Here's how the part is built. I have some questions about the finished solid (model axes, mm). Round coordinates to 2 decimals unless told otherwise and drop trailing zeros. Write each loop counter-clockwise with the first axis right and the second up, starting at its lowest first coordinate (ties: lowest second). Pieces come first, ordered by that corner, then holes. Notation, with made-up numbers: M 54.25,45.25 L 67.25,45.25 A24 cw 67.25,56.25 Z; hole C 49,54.5 d11. An arc over 180 degrees is marked long. Use one line per item in the form item = value. Start each with the question number.
Q1. I want a section at A-A on y = -6. List the corners of the cut face in (x, z) for me, and give its area (3 significant figures).
Q2. I want a section at C-C on x = 16. List the corners of the cut face in (y, z) for me, and give its area (3 significant figures).
Q3. I need wall thicknesses on line 1 along X through (y, z) = (-15.25, 0.25); line 2 along X through (y, z) = (-5.5, 0.8). Which ranges of each line are inside material? Lowest first, please. Write a range as from..to.
Q4. I want a section at D-D on z = 0.3. State how many separate pieces and enclosed holes the cut face has, and give its area (3 significant figures).
Q5. I'm going to push a flat-ended pin straight in: pin 1 Ø2.5 at (x, y) = (15.25, 15.25) entering from +Z. Where does the tip first touch, or does it pass through?
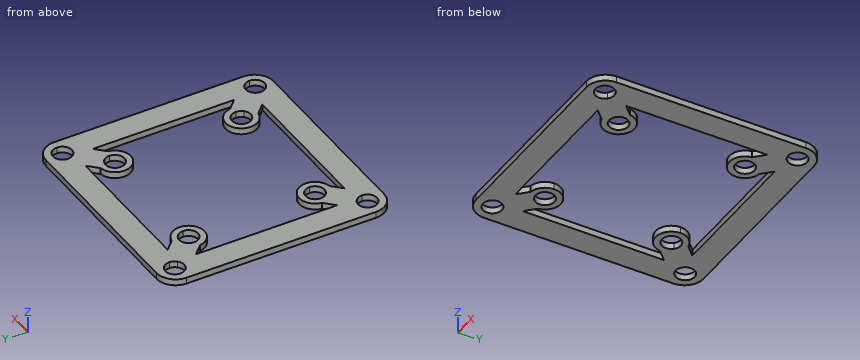
```python
from build123d import *

# Parameters (mm, degrees)
F1_DEPTH = 1


with BuildPart() as f1:
    # F0 (on Top) → F1 (new body)
    with BuildSketch(Plane.XY):
        with BuildLine():
            Line((15, 18), (-15, 18))
            ThreePointArc((-15, 18), (-17.1213203436, 17.1213203436), (-18, 15))
            Line((-18, 15), (-18, -15))
            ThreePointArc((-18, -15), (-17.1213203436, -17.1213203436), (-15, -18))
            Line((-15, -18), (15, -18))
            ThreePointArc((15, -18), (17.1213203436, -17.1213203436), (18, -15))
            Line((18, -15), (18, 15))
            ThreePointArc((18, 15), (17.1213203436, 17.1213203436), (15, 18))
        make_face()
        with BuildLine():
            ThreePointArc((-13.75, -15.25), (-16.6358192988, -15.8240251485), (-14.1893398282, -14.1893398282))
            ThreePointArc((-14.1893398282, -14.1893398282), (-13.8641807012, -14.6759748515), (-13.75, -15.25))
        make_face(mode=Mode.SUBTRACT)
        with BuildLine():
            ThreePointArc((16.75, -15.25), (14.6759748515, -16.6358192988), (14.1893398282, -14.1893398282))
            ThreePointArc((14.1893398282, -14.1893398282), (15.8240251485, -13.8641807012), (16.75, -15.25))
        make_face(mode=Mode.SUBTRACT)
        with BuildLine():
            ThreePointArc((-13.75, 15.25), (-13.8641807012, 14.6759748515), (-14.1893398282, 14.1893398282))
            ThreePointArc((-14.1893398282, 14.1893398282), (-16.6358192988, 15.8240251485), (-13.75, 15.25))
        make_face(mode=Mode.SUBTRACT)
        Polygon((-14, 11.1715728753), (-14, 14), (-11.1715728753, 14), (11.1715728753, 14), (14, 14), (14, 11.1715728753), (14, -11.1715728753), (14, -14), (11.1715728753, -14), (-11.1715728753, -14), (-14, -14), (-14, -11.1715728753), align=None, mode=Mode.SUBTRACT)
        with BuildLine():
            ThreePointArc((16.75, 15.25), (15.8240251485, 13.8641807012), (14.1893398282, 14.1893398282))
            ThreePointArc((14.1893398282, 14.1893398282), (14.6759748515, 16.6358192988), (16.75, 15.25))
        make_face(mode=Mode.SUBTRACT)
        with BuildLine():
            Line((-14, 14), (-11.767766953, 11.767766953))
            ThreePointArc((-11.767766953, 11.767766953), (-10.790569415, 12.3717082451), (-9.6464466094, 12.4748737342))
            Line((-9.6464466094, 12.4748737342), (-11.1715728753, 14))
            Line((-11.1715728753, 14), (-14, 14))
        make_face()
        with BuildLine():
            ThreePointArc((-12.4748737342, 9.6464466094), (-12.3717082451, 10.790569415), (-11.767766953, 11.767766953))
            Line((-11.767766953, 11.767766953), (-14, 14))
            Line((-14, 14), (-14, 11.1715728753))
            Line((-14, 11.1715728753), (-12.4748737342, 9.6464466094))
        make_face()
        with BuildLine():
            ThreePointArc((-9.6464466094, 12.4748737342), (-10.790569415, 12.3717082451), (-11.767766953, 11.767766953))
            ThreePointArc((-11.767766953, 11.767766953), (-12.3717082451, 10.790569415), (-12.4748737342, 9.6464466094))
            ThreePointArc((-12.4748737342, 9.6464466094), (-9.8227774498, 7.506289478), (-7.5, 10))
            ThreePointArc((-7.5, 10), (-8.1113651125, 11.6380043534), (-9.6464466094, 12.4748737342))
        make_face()
        with BuildLine():
            ThreePointArc((-11.0606601718, 11.0606601718), (-9.4259748515, 11.3858192988), (-8.5, 10))
            ThreePointArc((-8.5, 10), (-10.5740251485, 8.6141807012), (-11.0606601718, 11.0606601718))
        make_face(mode=Mode.SUBTRACT)
        with BuildLine():
            Line((14, 14), (11.1715728753, 14))
            Line((11.1715728753, 14), (9.6464466094, 12.4748737342))
            ThreePointArc((9.6464466094, 12.4748737342), (10.790569415, 12.3717082451), (11.767766953, 11.767766953))
            Line((11.767766953, 11.767766953), (14, 14))
        make_face()
        with BuildLine():
            Line((14, 11.1715728753), (14, 14))
            Line((14, 14), (11.767766953, 11.767766953))
            ThreePointArc((11.767766953, 11.767766953), (12.3096988313, 10.9567085809), (12.5, 10))
            ThreePointArc((12.5, 10), (12.493710522, 9.8227774498), (12.4748737342, 9.6464466094))
            Line((12.4748737342, 9.6464466094), (14, 11.1715728753))
        make_face()
        with BuildLine():
            ThreePointArc((11.767766953, 11.767766953), (10.790569415, 12.3717082451), (9.6464466094, 12.4748737342))
            ThreePointArc((9.6464466094, 12.4748737342), (8.232233047, 8.232233047), (12.4748737342, 9.6464466094))
            ThreePointArc((12.4748737342, 9.6464466094), (12.493710522, 9.8227774498), (12.5, 10))
            ThreePointArc((12.5, 10), (12.3096988313, 10.9567085809), (11.767766953, 11.767766953))
        make_face()
        with BuildLine():
            ThreePointArc((11.5, 10), (8.6141807012, 9.4259748515), (11.0606601718, 11.0606601718))
            ThreePointArc((11.0606601718, 11.0606601718), (11.3858192988, 10.5740251485), (11.5, 10))
        make_face(mode=Mode.SUBTRACT)
        with BuildLine():
            Line((14, -14), (14, -11.1715728753))
            Line((14, -11.1715728753), (12.4748737342, -9.6464466094))
            ThreePointArc((12.4748737342, -9.6464466094), (12.493710522, -9.8227774498), (12.5, -10))
            ThreePointArc((12.5, -10), (12.3096988313, -10.9567085809), (11.767766953, -11.767766953))
            Line((11.767766953, -11.767766953), (14, -14))
        make_face()
        with BuildLine():
            Line((9.6464466094, -12.4748737342), (11.1715728753, -14))
            Line((11.1715728753, -14), (14, -14))
            Line((14, -14), (11.767766953, -11.767766953))
            ThreePointArc((11.767766953, -11.767766953), (10.790569415, -12.3717082451), (9.6464466094, -12.4748737342))
        make_face()
        with BuildLine():
            ThreePointArc((12.5, -10), (12.493710522, -9.8227774498), (12.4748737342, -9.6464466094))
            ThreePointArc((12.4748737342, -9.6464466094), (8.232233047, -8.232233047), (9.6464466094, -12.4748737342))
            ThreePointArc((9.6464466094, -12.4748737342), (10.790569415, -12.3717082451), (11.767766953, -11.767766953))
            ThreePointArc((11.767766953, -11.767766953), (12.3096988313, -10.9567085809), (12.5, -10))
        make_face()
        with BuildLine():
            ThreePointArc((11.5, -10), (11.3858192988, -10.5740251485), (11.0606601718, -11.0606601718))
            ThreePointArc((11.0606601718, -11.0606601718), (8.6141807012, -9.4259748515), (11.5, -10))
        make_face(mode=Mode.SUBTRACT)
        with BuildLine():
            ThreePointArc((-7.5, -10), (-9.8227774498, -7.506289478), (-12.4748737342, -9.6464466094))
            ThreePointArc((-12.4748737342, -9.6464466094), (-12.3717082451, -10.790569415), (-11.767766953, -11.767766953))
            ThreePointArc((-11.767766953, -11.767766953), (-10.790569415, -12.3717082451), (-9.6464466094, -12.4748737342))
            ThreePointArc((-9.6464466094, -12.4748737342), (-8.1113651125, -11.6380043534), (-7.5, -10))
        make_face()
        with BuildLine():
            ThreePointArc((-8.5, -10), (-9.4259748515, -11.3858192988), (-11.0606601718, -11.0606601718))
            ThreePointArc((-11.0606601718, -11.0606601718), (-10.5740251485, -8.6141807012), (-8.5, -10))
        make_face(mode=Mode.SUBTRACT)
        with BuildLine():
            Line((-12.4748737342, -9.6464466094), (-14, -11.1715728753))
            Line((-14, -11.1715728753), (-14, -14))
            Line((-14, -14), (-11.767766953, -11.767766953))
            ThreePointArc((-11.767766953, -11.767766953), (-12.3717082451, -10.790569415), (-12.4748737342, -9.6464466094))
        make_face()
        with BuildLine():
            Line((-11.767766953, -11.767766953), (-14, -14))
            Line((-14, -14), (-11.1715728753, -14))
            Line((-11.1715728753, -14), (-9.6464466094, -12.4748737342))
            ThreePointArc((-9.6464466094, -12.4748737342), (-10.790569415, -12.3717082451), (-11.767766953, -11.767766953))
        make_face()
    extrude(amount=F1_DEPTH)


solid = f1.part
```
Reported:
q1.outline = M -18,0 L -14,0 L -14,1 L -18,1 Z; M 14,0 L 18,0 L 18,1 L 14,1 Z
q1.area = 8.00 mm^2
q2.outline = M -17.83,0 L -16.55,0 L -16.55,1 L -17.83,1 Z; M -13.95,0 L 13.95,0 L 13.95,1 L -13.95,1 Z; M 16.55,0 L 17.83,0 L 17.83,1 L 16.55,1 Z
q2.area = 30.5 mm^2
q3.line_1 = -17.99..-16.75, -13.75..13.75, 16.75..17.99
q3.line_2 = -18..-14, 14..18
q4.separate_pieces = 1
q4.enclosed_holes = 9
q4.area = 566 mm^2
q5.pin_1 = through
